Part model, mm, in its own coordinate system. Round coordinates to 2 decimals unless told otherwise and drop trailing zeros. Loops run counter-clockwise (first coordinate to the right, second up) from the corner with the lowest first, then second, coordinate; pieces in that order, holes last.
1) Band-saw the part on D-D, the plane x = 75. Write the cut outline in (y, z).
2) Band-saw the part on C-C, the plane z = 0.1. Write the cut outline in (x, y), then the cut area to 3 significant figures.
3) Band-saw the part on B-B, the plane x = 71.75. Write the cut outline in (y, z), then the cut area to 3 significant figures.
4) Band-saw the part on A-A, the plane y = 68. Write the cut outline in (x, z).
5) Probe line 1 (X direction, y = 63.75, z = 0.1); line 2 (X direction, y = 64, z = 0.15); line 3 (Y direction, x = 68.5, z = 0.15). List the from-to ranges inside material, lowest first.
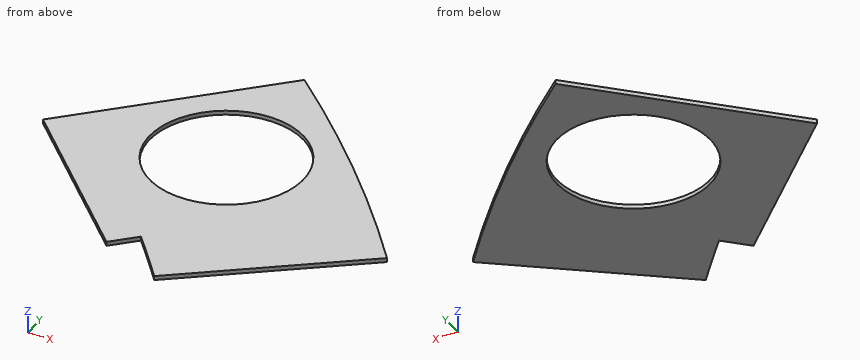
from build123d import *

# Parameters (mm, degrees)
BOSS_EXTRUDE1_DEPTH = 0.254
SKETCH2_R           = 4.699
CUT_EXTRUDE1_DEPTH  = 1.254
SKETCH3_W           = 2.54
SKETCH3_H           = 0.635
CUT_EXTRUDE2_DEPTH  = 1.254
SKETCH5_OUTSIDE_W   = 121.447
SKETCH5_OUTSIDE_H   = 109.618
CUT_EXTRUDE5_DEPTH  = 1.254


with BuildPart() as part:
    # Sketch1 → Boss-Extrude1 (new body)
    with BuildSketch(Plane.XY):
        with BuildLine():
            Line((67.21146711, 76.191723231), (8.696654013, 17.676910134))
            Line((8.696654013, 17.676910134), (7.228954972, 14.133571205))
            ThreePointArc((7.228954972, 14.133571205), (14.666587579, 6.075099489), (15.105587123, -4.88230096))
            Line((15.105587123, -4.88230096), (18.648926052, -6.35))
            Line((18.648926052, -6.35), (101.401368334, -6.35))
            ThreePointArc((101.401368334, -6.35), (93.866160503, 38.880636728), (67.21146711, 76.191723231))
        make_face()
        with BuildLine():
            Line((88.672924278, 6.35), (27.86051193, 6.35))
            ThreePointArc((27.86051193, 6.35), (26.399857642, 10.93517908), (24.190484974, 15.210228852))
            Line((24.190484974, 15.210228852), (67.191354125, 58.211098004))
            ThreePointArc((67.191354125, 58.211098004), (82.13289044, 34.020557137), (88.672924278, 6.35))
        make_face(mode=Mode.SUBTRACT)
    extrude(amount=BOSS_EXTRUDE1_DEPTH)

    # Sketch2 → Cut-Extrude1 (cut, through all)
    with BuildSketch(Plane.XY.offset(0.254)):
        with Locations((22.225, 0)):
            Circle(SKETCH2_R)
        with Locations((36.195, 0)):
            Circle(SKETCH2_R)
        with Locations((61.722, 0)):
            Circle(SKETCH2_R)
        with Locations((75.692, 0)):
            Circle(SKETCH2_R)
        with Locations((95.25, 0)):
            Circle(SKETCH2_R)
        with Locations((15.715448212, 15.715448212)):
            Circle(SKETCH2_R)
        with Locations((25.593729945, 25.593729945)):
            Circle(SKETCH2_R)
        with Locations((43.644044748, 43.644044748)):
            Circle(SKETCH2_R)
        with Locations((53.522326482, 53.522326482)):
            Circle(SKETCH2_R)
        with Locations((92.004434954, 24.652514046)):
            Circle(SKETCH2_R)
        with Locations((82.48891971, 47.625)):
            Circle(SKETCH2_R)
        with Locations((67.351920908, 67.351920908)):
            Circle(SKETCH2_R)
    extrude(amount=-CUT_EXTRUDE1_DEPTH, mode=Mode.SUBTRACT)

    # Sketch3 → Cut-Extrude2 (cut, through all)
    with BuildSketch(Plane.XY.offset(0.254)):
        Polygon((15.266435406, 24.246691527), (17.06248663, 26.042742751), (17.511499436, 25.593729945), (15.715448212, 23.797678721), align=None)
        Polygon((44.991083167, 53.971339288), (43.195031942, 52.175288063), (43.644044748, 51.726275257), (45.440095973, 53.522326482), align=None)
        with Locations((29.21, -6.0325)):
            Rectangle(SKETCH3_W, SKETCH3_H)
        with Locations((68.707, -6.0325)):
            Rectangle(SKETCH3_W, SKETCH3_H)
        Polygon((29.230733674, 38.210989795), (31.026784898, 40.007041019), (31.475797704, 39.558028213), (29.67974648, 37.761976989), align=None)
        Polygon((56.845021246, 65.825277367), (55.048970022, 64.029226143), (55.497982828, 63.580213337), (57.294034052, 65.376264561), align=None)
        with Locations((48.9585, -6.0325)):
            Rectangle(SKETCH3_W, SKETCH3_H)
        with Locations((85.471, -6.0325)):
            Rectangle(SKETCH3_W, SKETCH3_H)
        Polygon((99.935462164, 14.437711971), (100.266998693, 11.919442024), (101.526133667, 12.085210288), (101.194597138, 14.603480236), align=None)
        Polygon((93.765504959, 37.464305742), (94.938831965, 37.950313702), (93.966816047, 40.296967714), (92.793489041, 39.810959755), align=None)
        Polygon((79.327792988, 62.471156422), (80.874047017, 60.456038938), (81.88160576, 61.229165953), (80.33535173, 63.244283437), align=None)
        Polygon((13.593916116, 7.005422516), (14.565932035, 4.658768503), (15.739259041, 5.144776462), (14.767243123, 7.491430475), align=None)
    extrude(amount=-CUT_EXTRUDE2_DEPTH, mode=Mode.SUBTRACT)

    # Sketch5 outside → Cut-Extrude5 (cut, through all)
    with BuildSketch(Plane.XY.offset(0.254)):
        with Locations((54.4145, 34.921)):
            Rectangle(SKETCH5_OUTSIDE_W, SKETCH5_OUTSIDE_H)
        Polygon((55.946995634, 66.72330298), (68.504300263, 54.16599835), (81.410712434, 64.069436727), (67.351920908, 78.128228253), align=None, mode=Mode.SUBTRACT)
    extrude(amount=-CUT_EXTRUDE5_DEPTH, mode=Mode.SUBTRACT)


solid = part.part
Reported:
1. outline: (59.15, 0) - (68.54, 0) - (68.54, 0.25) - (59.15, 0.25) - close
2. outline: (56.85, 65.83) - (65.83, 56.85) - (67.19, 58.21) arc R88.9 cw to (69.75, 55.12) - (79.83, 62.85) arc R101.6 ccw to (67.21, 76.19) - close; hole circle Ø9.4 at (67.35, 67.35)
2. area: 180 mm2
3. outline: (56.66, 0) - (65.7, 0) - (65.7, 0.25) - (56.66, 0.25) - close; (69.01, 0) - (71.93, 0) - (71.93, 0.25) - (69.01, 0.25) - close
3. area: 3.04 mm2
4. outline: (59.02, 0) - (62.7, 0) - (62.7, 0.25) - (59.02, 0.25) - close; (72.01, 0) - (75.49, 0) - (75.49, 0.25) - (72.01, 0.25) - close
5. line 1: x = 58.92 to 64.33, 70.37 to 79.11
5. line 2: x = 58.67 to 64.06, 70.65 to 78.91
5. line 3: y = 56.67 to 62.8, 71.91 to 75.04
